The listing builds one solid part. Answer for the finished solid, in the listing's coordinates (mm). A direction names the side the tool comes from. Round coordinates to 2 decimals unless told otherwise and drop trailing zeros. Order: outer loops, then holes, each group sorted by start corner. A loop starts at its lowest first (then second) coordinate and runs counter-clockwise, first axis right, second up. Notation, with made-up numbers: (82.5, -8.5) -> (110.5, -8.5) arc R27 cw to (110.5, 13.5) -> close; hole circle Ø4 at (-29, 16). An arc over 180 degrees is marked (long way). Answer in a Markdown table with one row per item. Add a question column.
```python
from build123d import *

# Parameters (mm, degrees)
SKETCH1_W           = 110
SKETCH1_H           = 112
BOSS_EXTRUDE1_DEPTH = 3
SKETCH2_R           = 9
SKETCH2_W           = 70
SKETCH2_H           = 22
CUT_EXTRUDE1_DEPTH  = 79.549347547
CUT_EXTRUDE2_DEPTH  = 79.549347547
CHAMFER1_SIZE       = 2
SKETCH4_R           = 4
BOSS_EXTRUDE2_DEPTH = 4
SKETCH5_R           = 1.75
CUT_EXTRUDE3_DEPTH  = 79.803553219
FILLET1_R           = 3
SKETCH6_R           = 2.2
CUT_EXTRUDE4_DEPTH  = 79.593892893


with BuildPart() as part:
    # Sketch1 → Boss-Extrude1 (new body)
    with BuildSketch(Plane.XY):
        Rectangle(SKETCH1_W, SKETCH1_H)
    extrude(amount=BOSS_EXTRUDE1_DEPTH)

    # Sketch2 → Cut-Extrude1 (cut, through all)
    with BuildSketch(Plane.XY.offset(3)):
        with Locations((0, 12)):
            Circle(SKETCH2_R)
        with Locations((0, -45)):
            Rectangle(SKETCH2_W, SKETCH2_H)
    extrude(amount=-CUT_EXTRUDE1_DEPTH, mode=Mode.SUBTRACT)

    # Sketch3 → Cut-Extrude2 (cut, through all)
    with BuildSketch(Plane.XY.offset(3)):
        with BuildLine():
            Line((-33, 46), (-5, 46))
            Line((-5, 46), (-5, 32))
            ThreePointArc((-5, 32), (-9.393398282, 21.393398282), (-20, 17))
            Line((-20, 17), (-45, 17))
            Line((-45, 17), (-45, 34))
            Line((-45, 34), (-33, 46))
        make_face()
        with BuildLine():
            Line((45, 34), (33, 46))
            Line((33, 46), (5, 46))
            Line((5, 46), (5, 32))
            ThreePointArc((5, 32), (9.393398282, 21.393398282), (20, 17))
            Line((20, 17), (45, 17))
            Line((45, 17), (45, 34))
        make_face()
        with BuildLine():
            Line((33, -22), (5, -22))
            Line((5, -22), (5, -8))
            ThreePointArc((5, -8), (9.393398282, 2.606601718), (20, 7))
            Line((20, 7), (45, 7))
            Line((45, 7), (45, -10))
            Line((45, -10), (33, -22))
        make_face()
        with BuildLine():
            Line((-45, -10), (-33, -22))
            Line((-33, -22), (-5, -22))
            Line((-5, -22), (-5, -8))
            ThreePointArc((-5, -8), (-9.393398282, 2.606601718), (-20, 7))
            Line((-20, 7), (-45, 7))
            Line((-45, 7), (-45, -10))
        make_face()
    extrude(amount=-CUT_EXTRUDE2_DEPTH, mode=Mode.SUBTRACT)

    # Chamfer1
    chamfer1_edges = [part.edges().sort_by_distance(p)[0] for p in [
        (-9, 12, 3),
    ]]
    chamfer(chamfer1_edges, length=CHAMFER1_SIZE)

    # Sketch4 → Boss-Extrude2 (add)
    with BuildSketch(Plane.XY.offset(3)):
        with Locations(Location((-50, -29, 0), (0, 0, 180))):
            Circle(SKETCH4_R)
        with Locations(Location((50, -29, 0), (0, 0, 180))):
            Circle(SKETCH4_R)
        with Locations(Location((50, 51, 0), (0, 0, 180))):
            Circle(SKETCH4_R)
        with Locations(Location((-50, 51, 0), (0, 0, 180))):
            Circle(SKETCH4_R)
    extrude(amount=BOSS_EXTRUDE2_DEPTH)

    # Sketch5 → Cut-Extrude3 (cut, through all)
    with BuildSketch(Plane.XY.offset(7)):
        with Locations((-50, 51)):
            Circle(SKETCH5_R)
        with Locations((50, 51)):
            Circle(SKETCH5_R)
        with Locations((50, -29)):
            Circle(SKETCH5_R)
        with Locations((-50, -29)):
            Circle(SKETCH5_R)
    extrude(amount=-CUT_EXTRUDE3_DEPTH, mode=Mode.SUBTRACT)

    # Fillet1
    fillet1_edges = [part.edges().sort_by_distance(p)[0] for p in [
        (-35, -56, 1.5),
        (35, -56, 1.5),
        (-55, 56, 1.5),
        (55, 56, 1.5),
        (55, -56, 1.5),
        (-55, -56, 1.5),
    ]]
    fillet(fillet1_edges, radius=FILLET1_R)

    # Sketch6 → Cut-Extrude4 (cut, through all)
    with BuildSketch(Plane.XY.offset(3)):
        with Locations((-45, -46)):
            Circle(SKETCH6_R)
        with Locations((45, -46)):
            Circle(SKETCH6_R)
    extrude(amount=-CUT_EXTRUDE4_DEPTH, mode=Mode.SUBTRACT)


solid = part.part
```
1. The part is cut by section C-C (x = 24). Give the vertices of the cut face in (y, z).
2. The part is cut by section D-D (y = -6). Give the vertices of the cut face in (x, z), then the cut area to 3 significant figures.
3. The mould has two halves that part along X. Classify faces 5 (the flat face through (-55, -1, 1)), 6 (the flat face through (45, -56, 1)), 7 (the flat face through (-45, -1, 2)): released by +X, released by -X, zero draft, split by the parting line, or undercut.
4. For faces 1 (the flat face through (49, 53, 7)), 2 (the cylindrical face through (-46.8, 53.4, 5)), 3 (the flat face through (35, -44, 2)), 4 (the flat face through (5, -15, 2)), determine the directions among +Z, -Z, +X, -X, +Y, -Y from which every point of the face is accessible in a straight line to the end or side of a thin tool.
5. Each of these flat-tipped pins is pushed along its axis until it touches: pin 1 (10 mm diameter, centred on x = 5.5, y = -6.5, fed in from +Z); pin 2 (1.5 mm diameter, centred on x = -37, z = 2, fed in from -Y); pin 3 (0.9 mm diameter, centred on x = -19, z = 2, fed in from -Y). Where does it stop, or does it pass through?
6. The part is cut by section A-A (y = 12). Give the vertices of the cut face in (x, z).
7. Straight lines are drawn through the part: line 1 along Y through (x, z) = (-50, 3.25); line 2 along Y through (x, z) = (-50, 2.5); line 3 along Y through (x, z) = (-12, 1.5). For each, find the intervals that lie inside material, in ascending order.
8. The part is cut by section B-B (z = 4.25). Give the vertices of the cut face in (x, y).
Report:
| question | item | result |
|---|---|---|
| 1 | outline | (-34, 0) -> (-22, 0) -> (-22, 3) -> (-34, 3) -> close; (7, 0) -> (17, 0) -> (17, 3) -> (7, 3) -> close; (46, 0) -> (56, 0) -> (56, 3) -> (46, 3) -> close |
| 2 | outline | (-55, 0) -> (-45, 0) -> (-45, 3) -> (-55, 3) -> close; (-5.13, 0) -> (5.13, 0) -> (5.13, 3) -> (-5.13, 3) -> close; (45, 0) -> (55, 0) -> (55, 3) -> (45, 3) -> close |
| 2 | area | 90.8 mm^2 |
| 3 | face 5 | released by -X |
| 3 | face 6 | zero draft |
| 3 | face 7 | undercut |
| 4 | face 1 | +Z, +X, -X, +Y, -Y |
| 4 | face 2 | +Z |
| 4 | face 3 | +Z, -Z, -Y |
| 4 | face 4 | +Z, -Z |
| 5 | pin 1 | stops at z = 3 |
| 5 | pin 2 | stops at y = -55.99 |
| 5 | pin 3 | stops at y = -34 |
| 6 | outline | (-55, 0) -> (-9, 0) -> (-9, 1) -> (-11, 3) -> (-55, 3) -> close; (9, 0) -> (55, 0) -> (55, 3) -> (11, 3) -> (9, 1) -> close |
| 7 | line 1 | y = -33 to -30.75, -27.25 to -25, 47 to 49.25, 52.75 to 55 |
| 7 | line 2 | y = -56 to -30.75, -27.25 to 49.25, 52.75 to 56 |
| 7 | line 3 | y = -34 to -22, 4.69 to 19.31, 46 to 56 |
| 8 | outline | circle Ø8 at (-50, -29); circle Ø8 at (-50, 51); circle Ø8 at (50, -29); circle Ø8 at (50, 51); hole circle Ø3.5 at (-50, -29); hole circle Ø3.5 at (-50, 51); hole circle Ø3.5 at (50, -29); hole circle Ø3.5 at (50, 51) |
